Autodesk Inventor part; units mm, degrees
ref_plane "Work Plane1" through (0, 300, 0) normal (0, -1, 0) x (1, 0, 0)
ref_plane "YZ Plane" through (0, 0, 0) normal (1, 0, 0) x (0, 1, 0)
ref_plane "XZ Plane" through (0, 0, 0) normal (0, 1, 0) x (-1, 0, 0)
sketch "Sketch1" plane through (0, 0, 0) normal (0, 1, 0) x (-1, 0, 0)
  circle A0 centre (0, 0) radius 8
  dimension "d0" = 16
extrude "Extrusion1" add sketch "Sketch1" along normal blind 600
sketch "Sketch2" plane through (0, 0, 0) normal (0, -1, 0) x (1, 0, 0)
  circle A0 centre (0, 0) radius 3.5
  dimension "d7" = 7
extrude "Extrusion2" cut sketch "Sketch2" against normal blind 10
ref_plane "Work Plane1" through (0, 300, 0) normal (0, -1, 0) x (1, 0, 0)
mirror "Mirror1" about plane through (0, 300, 0) normal (0, -1, 0) of "Extrusion2"
properties part number "ScrewDriver" material "Aluminum 6061"
Work out the finished part from the listing and answer in its coordinate system (mm). Give positions to 0.01 mm unless a question says otherwise; leave off trailing zeros. Order: outer loops, then holes, each group sorted by start corner. A loop starts at its lowest first (then second) coordinate and runs counter-clockwise, first axis right, second up. Notation, with made-up numbers: M 29,-21.5 L 37,-21.5 A13 cw 37,0.5 Z; hole C 61,2.25 d2. An arc over 180 degrees is marked long. Return JSON: item names as keys, results as strings.
Q1. Find the intervals of material crossed by line 1 along Z through (x, y) = (0, 597); line 2 along X through (y, z) = (528.5, 1.25); line 3 along Y through (x, z) = (-1, -2), in increasing order. Write a range as [from, to].
Answer below:
{"line 1": "z = [-8, -3.5], [3.5, 8]", "line 2": "x = [-7.9, 7.9]", "line 3": "y = [10, 590]"}
Q2. Find section B-B, the plane y = 205.5. Write down the section's boundary in (x, z), and give its area (3 significant figures).
Answer below:
{"outline": "C 0,0 d16", "area": "201 mm^2"}
Q3. Each of these flat-tipped pins is pushed along its axis until it touches: pin 1 (6.5 mm diameter, centred on x = 0, z = 0, fed in from -Y); pin 2 (6 mm diameter, centred on y = 133.5, z = 1.5, fed in from -X); pin 3 (8 mm diameter, centred on x = -4.5, y = 478, fed in from -Z); pin 4 (1.5 mm diameter, centred on y = 492.5, z = 5.5, fed in from +X). Where does it stop, or does it pass through?
Answer below:
{"pin 1": "stops at y = 10", "pin 2": "stops at x = -8", "pin 3": "stops at z = -7.98", "pin 4": "stops at x = 6.44"}
Q4. Find section A-A, the plane x = -1. Write down the section's boundary in (y, z), and give its area (3 significant figures).
Answer below:
{"outline": "M 0,-7.94 L 600,-7.94 L 600,-3.35 L 590,-3.35 L 590,3.35 L 600,3.35 L 600,7.94 L 0,7.94 L 0,3.35 L 10,3.35 L 10,-3.35 L 0,-3.35 Z", "area": "9,390 mm^2"}
